Geometry: final body of the model. Coordinates: model frame, mm. A direction names the side the tool comes from. Round coordinates to 2 decimals unless told otherwise and drop trailing zeros. Order: outer loops, then holes, each group sorted by start corner. A loop starts at its lowest first (then second) coordinate and runs counter-clockwise, first axis right, second up. Notation, with made-up numbers: M 24.25,67 L 50.25,67 A11 cw 50.25,75 Z; hole C 17.5,42 d4. An arc over 180 degrees is marked long. Return JSON: item names as keys, results as strings. Group by question number.
Q1. Cut plane A-A on z = 0. Output: boundary loops of the cut face in (x, y).
Q2. Access query for faces 1 (the face through (1, 0, 1)), 2 (the face through (0, 1.5, 0)), 3 (the face through (0, 12, 2)). Directions: +Z, -Z, +X, -X, +Y, -Y. A direction counts if a zero-diameter tool reaches every point of the face in a straight line with its end or side. Return the directions, or none.
Q3. Mould query, pull axis X, two halves, no side actions, for faces 4 (the face through (0.5, 0.7, -1.5)), 5 (the face through (-2.5, 1.06, 1.917)), 6 (the face through (0, 22.15, 0)). Classes: released by +X, released by -X, zero draft, split by the parting line, or undercut.
Q4. Cut plane B-B on x = 0. Output: boundary loops of the cut face in (y, z).
Q5. Contact query for flat-ended pins moving along their axis: pin 1 (0.8 mm diameter, centred on y = 0.5, z = 1.5, fed in from +X); pin 2 (1.1 mm diameter, centred on x = -1.5, y = 0.5, fed in from -Z); pin 3 (0.8 mm diameter, centred on x = 1.5, y = 1, fed in from +Z). Output: stop coordinate, or through.
Q6. Cut plane D-D on x = -2.5. Output: boundary loops of the cut face in (y, z).
Q7. Ray query, probe 1 along Y at (x, z) = (-1.5, 2.25); probe 2 along Z at (x, y) = (0, 21); probe 3 along X at (y, z) = (4, -1). Return the intervals inside material, ascending.
Q8. Cut plane C-C on y = 11.5. Output: boundary loops of the cut face in (x, z).
```python
from build123d import *

# Parameters (mm, degrees)
SKETCH_1_R          = 3.15
EXTRUDE_1_DEPTH     = 2.15
SKETCH_2_R          = 2
EXTRUDE_2_DEPTH     = 20
CUT_EXTRUDE_1_DEPTH = 1.5


with BuildPart() as part:
    # 草图1 → 凸台-拉伸1 (new body)
    with BuildSketch(Plane(origin=(0, 0, 0), x_dir=(1, 0, 0), z_dir=(0, 1, 0))):
        Circle(SKETCH_1_R)
    extrude(amount=EXTRUDE_1_DEPTH)

    # 草图2 → 凸台-拉伸2 (add)
    with BuildSketch(Plane(origin=(0, 2.15, 0), x_dir=(1, 0, 0), z_dir=(0, 1, 0))):
        Circle(SKETCH_2_R)
    extrude(amount=EXTRUDE_2_DEPTH)

    # 草图3 → 切除-拉伸1 (cut)
    with BuildSketch(Plane.XZ):
        with BuildLine():
            Line((-0.5, 1), (-0.5, 2))
            Line((-0.5, 2), (0.5, 2))
            Line((0.5, 2), (0.5, 1))
            ThreePointArc((0.5, 1), (0.646446609, 0.646446609), (1, 0.5))
            Line((1, 0.5), (2, 0.5))
            Line((2, 0.5), (2, -0.5))
            Line((2, -0.5), (1, -0.5))
            ThreePointArc((1, -0.5), (0.646446609, -0.646446609), (0.5, -1))
            Line((0.5, -1), (0.5, -2))
            Line((0.5, -2), (-0.5, -2))
            Line((-0.5, -2), (-0.5, -1))
            ThreePointArc((-0.5, -1), (-0.646446609, -0.646446609), (-1, -0.5))
            Line((-1, -0.5), (-2, -0.5))
            Line((-2, -0.5), (-2, 0.5))
            Line((-2, 0.5), (-1, 0.5))
            ThreePointArc((-1, 0.5), (-0.646446609, 0.646446609), (-0.5, 1))
        make_face()
    extrude(amount=-CUT_EXTRUDE_1_DEPTH, mode=Mode.SUBTRACT)


solid = part.part
```
Result sheet:
{
 "1": {"outline": "M -3.15,0 L -2,0 L -2,1.5 L 2,1.5 L 2,0 L 3.15,0 L 3.15,2.15 L 2,2.15 L 2,22.15 L -2,22.15 L -2,2.15 L -3.15,2.15 Z"},
 "2": {"face 1": "+Z, -Z, +X, -X, -Y", "face 2": "-Y", "face 3": "+Y"},
 "3": {"face 4": "undercut", "face 5": "split by the parting line", "face 6": "zero draft"},
 "4": {"outline": "M 0,-3.15 L 2.15,-3.15 L 2.15,-2 L 22.15,-2 L 22.15,2 L 2.15,2 L 2.15,3.15 L 0,3.15 L 0,2 L 1.5,2 L 1.5,-2 L 0,-2 Z"},
 "5": {"pin 1": "stops at x = 2.95", "pin 2": "stops at z = -3", "pin 3": "stops at z = 2.95"},
 "6": {"outline": "M 0,-1.92 L 2.15,-1.92 L 2.15,1.92 L 0,1.92 Z"},
 "7": {"probe 1": "y = 0 to 2.15", "probe 2": "z = -2 to 2", "probe 3": "x = -1.73 to 1.73"},
 "8": {"outline": "C 0,0 d4"}
}
